CAD build for the part. Positions are in the model's coordinates, mm. A direction names the side the tool comes from. Give positions to 0.01 mm unless a question says otherwise; leave off trailing zeros. Write each loop counter-clockwise with the first axis right and the second up, starting at its lowest first coordinate (ties: lowest second). Pieces come first, ordered by that corner, then holes. Notation, with made-up numbers: M -14,19.25 L 44,19.25 A10 ccw 44,36.25 Z; hole C 87.25,82 d8. An arc over 180 degrees is marked long. One line per question, with ' | ' between items. Start each with the question number.
1. Cut at D-D, the plane y = 1.75. Write the cut outline in (x, z) (3 decimals), then the cut area to 3 significant figures.
2. Pull direction Z, two halves, no side cores. Call faces 1 (the face through (-3.3, 10.7, -0.7)), 2 (the face through (0.9, 13.49, 2.86)): released by +Z, released by -Z, zero draft, split by the parting line, or undercut.
3. Cut at C-C, the plane y = 13.25. Write the cut outline in (x, z) (3 decimals), then the cut area to 3 significant figures.
4. Which spindle directions (+Z, -Z, +X, -X, +Y, -Y) get a long thin tool onto all of the face, cutting with end or side? Do faces 3 (the face through (-1.978, 1.972, 2.579)), 4 (the face through (-1.39, 3.82, -3.35)). Say none if no direction does.
5. Flat gauge pin, fed straight in: pin 1 (4 mm diameter, centred on y = 3, z = -2.5, fed in from -X). Where does the tip first touch, or does it go through?
6. Wall check: L1, parallel to Z at x = 0, y = 13.45 (3 decimals); L2, parallel to X at y = 1.75, z = 0 (3 decimals). Give the ranges that are in metal, low to high.
```python
from build123d import *

# Parameters (mm, degrees)
SKETCH1_R           = 3.375
SKETCH1_R_2         = 3
BOSS_EXTRUDE1_DEPTH = 14
SKETCH2_R           = 3.625
SKETCH2_R_2         = 3
BOSS_EXTRUDE2_DEPTH = 8
FILLET1_R           = 0.25
BOSS_EXTRUDE3_START = -0.5
SKETCH3_R           = 3.375
SKETCH3_R_2         = 3
BOSS_EXTRUDE3_DEPTH = 0.5
FILLET2_R           = 0.5
SKETCH4_R           = 3.25
CUT_EXTRUDE1_DEPTH  = 4
SKETCH5_R           = 3.25
CUT_EXTRUDE2_DEPTH  = 1


# Some blends are built 0.0001 mm under size
with BuildPart() as part:
    # Sketch1 → Boss-Extrude1 (new body)
    with BuildSketch(Plane(origin=(0, 0, 0), x_dir=(1, 0, 0), z_dir=(0, 1, 0))):
        with Locations(Location((0, 0, 0), (0, 0, 270))):
            Circle(SKETCH1_R)
        with Locations(Location((0, 0, 0), (0, 0, 270))):
            Circle(SKETCH1_R_2, mode=Mode.SUBTRACT)
    extrude(amount=BOSS_EXTRUDE1_DEPTH)

    # Sketch2 → Boss-Extrude2 (add)
    with BuildSketch(Plane.XZ):
        with Locations(Location((0, 0, 0), (0, 0, 270))):
            Circle(SKETCH2_R)
        with Locations(Location((0, 0, 0), (0, 0, 90))):
            Circle(SKETCH2_R_2, mode=Mode.SUBTRACT)
    extrude(amount=-BOSS_EXTRUDE2_DEPTH)

    # Fillet1
    fillet1_edges = [part.edges().sort_by_distance(p)[0] for p in [
        (0, 8, 3.625),
    ]]
    fillet(fillet1_edges, radius=FILLET1_R - 0.0001)  # a hair under: the kernel refuses the full size

    # Sketch3 → Boss-Extrude3 (add)
    with BuildSketch(Plane(origin=(0, 14, 0), x_dir=(1, 0, 0), z_dir=(0, 1, 0)).offset(BOSS_EXTRUDE3_START)):
        with Locations(Location((0, 0, 0), (0, 0, 90))):
            Circle(SKETCH3_R)
        with Locations(Location((0, 0, 0), (0, 0, 270))):
            Circle(SKETCH3_R_2, mode=Mode.SUBTRACT)
    extrude(amount=BOSS_EXTRUDE3_DEPTH)

    # Fillet2
    # the kernel refuses this fillet: 0.5 mm, written as the material it takes off along each edge
    with BuildSketch(Plane(origin=(0, 14, 0), x_dir=(0, 0, 1), z_dir=(1, 0, 0))) as fillet2_piece_1:
        with BuildLine():
            CenterArc((2.875, 0.484122918), FILLET2_R, 284.477512186, 75.522487814)
            Line((3.375, 0.484122918), (3.385, 0.484122918))
            Line((3.385, 0.484122918), (3.385, 0))
            Line((3.385, 0), (3.375, -0.01))
            ThreePointArc((3.375, -0.01), (3.1875, -0.01), (3.0025, -0.009682458))
            Line((3.0025, -0.009682458), (3, 0))
        make_face()
    revolve(axis=Axis((0, 14, 0), (0, -1, 0)), mode=Mode.SUBTRACT)

    # Sketch4 → Cut-Extrude1 (cut)
    with BuildSketch(Plane.XZ):
        with Locations(Location((0, 0, 0), (0, 0, 270))):
            Circle(SKETCH4_R)
    extrude(amount=-CUT_EXTRUDE1_DEPTH, mode=Mode.SUBTRACT)

    # Sketch5 → Cut-Extrude2 (cut)
    with BuildSketch(Plane(origin=(0, 12, 0), x_dir=(-1, 0, 0), z_dir=(0, -1, 0))):
        with Locations(Location((0, 0, 0), (0, 0, 90))):
            Circle(SKETCH5_R)
    extrude(amount=-CUT_EXTRUDE2_DEPTH, mode=Mode.SUBTRACT)


solid = part.part
```
Here are the results:
1) outline: C 0,0 d7.25; hole C 0,0 d6.5 | area: 8.10 mm^2
2) face 1: split by the parting line | face 2: undercut
3) outline: C 0,0 d6.75; hole C 0,0 d6 | area: 7.51 mm^2
4) face 3: -Y | face 4: +Y, -Y
5) pin 1: x = -3.59
6) L1: -3.375 to -3, 3 to 3.375 | L2: -3.625 to -3.25, 3.25 to 3.625
